```python
from build123d import *

# Parameters (mm, degrees)
SKETCH1_W                = 127
SKETCH1_H                = 127
SKETCH1_R                = 38.1
BOSS_EXTRUDE1_DEPTH      = 76.2
SKETCH2_R                = 6.35
CUT_EXTRUDE1_DEPTH       = 25.4
SKETCH3_R                = 63.5
SKETCH3_R_2              = 38.1
BOSS_EXTRUDE2_DEPTH      = 12.7
SKETCH4_W                = 12.7
SKETCH4_H                = 20.32
BOSS_EXTRUDE3_DEPTH      = 25.4
FILLET1_R                = 2.54
FILLET1_OF_MIRROR2_R     = 2.54
SKETCH5_W                = 76.2
SKETCH5_H                = 50.8
CUT_EXTRUDE3_DEPTH       = 10.16
FILLET2_R                = 7.62
SKETCH6_R                = 38.1
SKETCH6_R_2              = 31.75
BOSS_EXTRUDE4_DEPTH      = 25.4
BOSS_EXTRUDE4_DEPTH_BACK = 25.4


with BuildPart() as part:
    # Sketch1 → Boss-Extrude1 (new body)
    with BuildSketch(Plane(origin=(0, 0, 0), x_dir=(1, 0, 0), z_dir=(0, 1, 0))):
        Rectangle(SKETCH1_W, SKETCH1_H)
        Circle(SKETCH1_R, mode=Mode.SUBTRACT)
    extrude(amount=BOSS_EXTRUDE1_DEPTH)

    # Sketch2 → Cut-Extrude1 (cut)
    with BuildSketch(Plane.ZY.offset(63.5)):
        with Locations((-44.45, 57.15)):
            Circle(SKETCH2_R)
        with Locations((-44.45, 19.05)):
            Circle(SKETCH2_R)
        with Locations((44.45, 57.15)):
            Circle(SKETCH2_R)
        with Locations((44.45, 19.05)):
            Circle(SKETCH2_R)
    cut_extrude1 = extrude(amount=-CUT_EXTRUDE1_DEPTH, mode=Mode.SUBTRACT)

    # Mirror1: Cut-Extrude1 across plane
    add(cut_extrude1.mirror(Plane(origin=(0, 0, 0), x_dir=(0, 0, 1), z_dir=(1, 0, 0))), mode=Mode.SUBTRACT)

    # Sketch3 → Boss-Extrude2 (add)
    with BuildSketch(Plane.XZ):
        Circle(SKETCH3_R)
        Circle(SKETCH3_R_2, mode=Mode.SUBTRACT)
    extrude(amount=BOSS_EXTRUDE2_DEPTH)

    # Sketch4 → Boss-Extrude3 (add)
    with BuildSketch(Plane.XY.offset(63.5)):
        with Locations((-69.85, 38.1)):
            Rectangle(SKETCH4_W, SKETCH4_H)
        with Locations((69.85, 38.1)):
            Rectangle(SKETCH4_W, SKETCH4_H)
    boss_extrude3 = extrude(amount=-BOSS_EXTRUDE3_DEPTH)

    # Fillet1
    fillet1_edges = [part.edges().sort_by_distance(p)[0] for p in [
        (-69.85, 27.94, 38.1),
        (-69.85, 48.26, 38.1),
        (-69.85, 48.26, 63.5),
        (-69.85, 27.94, 63.5),
        (69.85, 48.26, 38.1),
        (69.85, 27.94, 38.1),
        (69.85, 27.94, 63.5),
        (69.85, 48.26, 63.5),
    ]]
    fillet(fillet1_edges, radius=FILLET1_R)

    # Mirror2: Boss-Extrude3 across plane
    add(boss_extrude3.mirror(Plane.XY))

    # Fillet1 of Mirror2
    fillet1_of_mirror2_edges = [part.edges().sort_by_distance(p)[0] for p in [
        (-69.85, 27.94, -38.1),
        (-69.85, 48.26, -38.1),
        (-69.85, 48.26, -63.5),
        (-69.85, 27.94, -63.5),
        (69.85, 48.26, -38.1),
        (69.85, 27.94, -38.1),
        (69.85, 27.94, -63.5),
        (69.85, 48.26, -63.5),
    ]]
    fillet(fillet1_of_mirror2_edges, radius=FILLET1_OF_MIRROR2_R)

    # Sketch5 → Cut-Extrude3 (cut)
    with BuildSketch(Plane(origin=(0, 0, 63.5), x_dir=(-1, 0, 0), z_dir=(0, 0, -1))):
        with Locations((0, 38.1)):
            Rectangle(SKETCH5_W, SKETCH5_H)
    extrude(amount=CUT_EXTRUDE3_DEPTH, mode=Mode.SUBTRACT)

    # Fillet2
    fillet2_edges = [part.edges().sort_by_distance(p)[0] for p in [
        (38.1, 63.5, 58.42),
        (38.1, 12.7, 58.42),
        (-38.1, 12.7, 58.42),
        (-38.1, 63.5, 58.42),
    ]]
    fillet(fillet2_edges, radius=FILLET2_R)

    # Sketch6 → Boss-Extrude4 (add, two sides)
    with BuildSketch(Plane(origin=(0, 31.75, 0), x_dir=(-1, 0, 0), z_dir=(0, -1, 0))) as boss_extrude4_sk:
        Circle(SKETCH6_R)
        Circle(SKETCH6_R_2, mode=Mode.SUBTRACT)
    extrude(amount=BOSS_EXTRUDE4_DEPTH)
    extrude(boss_extrude4_sk.sketch, amount=-BOSS_EXTRUDE4_DEPTH_BACK)


solid = part.part
```
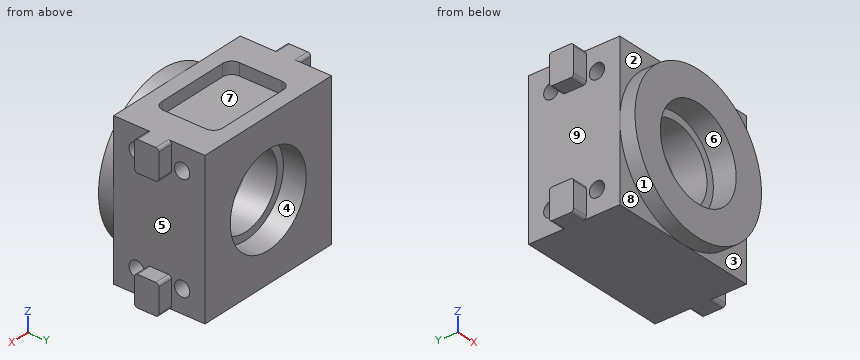
Check sheet for the modelled part. Datum: model origin and axes. Units: mm. Face numbers are marked on the shaded views. A direction names the side the tool comes from. Coordinates: 2 decimals unless noted, no trailing zeros. Loops run counter-clockwise (first coordinate to the right, second up) from the corner with the lowest first, then second, coordinate; pieces in that order, holes last. Notation, with made-up numbers: M -1.5,84.5 L 52.5,84.5 A23 cw 52.5,94.5 Z; hole C 4,-6.5 d4. An arc over 180 degrees is marked long. Answer as a JSON object with one key per item and string values.
1. Sectioned sample at D-D on x = -40.5. Record the cut outline in (y, z), and give its area (3 significant figures).
Outcome:
{"outline": "M -12.7,-48.91 L 0,-48.91 L 0,-63.5 L 76.2,-63.5 L 76.2,63.5 L 0,63.5 L 0,48.91 L -12.7,48.91 Z; hole C 19.05,-44.45 d12.7; hole C 19.05,44.45 d12.7; hole C 57.15,-44.45 d12.7; hole C 57.15,44.45 d12.7", "area": "10,400 mm²"}
2. Access from +Z, -Z, +X, -X, +Y, -Y to the whole of each face (thin tool, end or side, straight path). Record for the marked faces 1, 2, 3, 4 and 5.
Outcome:
{"face 1": "-Y", "face 2": "+Z, -X, -Y", "face 3": "-Z, +X, -Y", "face 4": "+Y", "face 5": "+X"}
3. Sectioned sample at A-A on z = -12. Record the cut outline in (x, y), and give its area (3 significant figures).
Outcome:
{"outline": "M -63.5,0 L -62.36,0 L -62.36,-12.7 L -36.16,-12.7 L -36.16,6.35 L -29.39,6.35 L -29.39,57.15 L -36.16,57.15 L -36.16,76.2 L -63.5,76.2 Z; M 29.39,6.35 L 36.16,6.35 L 36.16,-12.7 L 62.36,-12.7 L 62.36,0 L 63.5,0 L 63.5,76.2 L 36.16,76.2 L 36.16,57.15 L 29.39,57.15 Z", "area": "5,520 mm²"}
4. Sectioned sample at B-B on x = 44.5. Record the cut outline in (y, z), and give its area (3 significant figures).
Outcome:
{"outline": "M -12.7,-45.3 L 0,-45.3 L 0,-63.5 L 76.2,-63.5 L 76.2,63.5 L 0,63.5 L 0,45.3 L -12.7,45.3 Z; hole C 19.05,-44.45 d12.7; hole C 19.05,44.45 d12.7; hole C 57.15,-44.45 d12.7; hole C 57.15,44.45 d12.7", "area": "10,300 mm²"}
5. Scan lines: L1, parallel to Y at x = -46.75, z = -44.45; L2, parallel to Z at x = -49, y = 19; L3, parallel to X at y = 50, z = 0. Record each from-to range of solid material in increasing order. Write a range as from..to.
Outcome:
{"L1": "0..12.7, 25.4..50.8, 63.5..76.2", "L2": "-63.5..-50.8, -38.1..38.1, 50.8..63.5", "L3": "-63.5..-31.75, 31.75..63.5"}
6. Release check for a two-part mould opening along Z. For the marked faces 6, 7, 8 and 9 record: pulls with the +Z half, pulls with the -Z half, needs draft (parallel to the pull), parting line crosses it, or undercut.
Outcome:
{"face 6": "undercut", "face 7": "pulls with the +Z half", "face 8": "needs draft", "face 9": "undercut"}
7. Depth check by flat-ended pin: P1, Ø7.5, axis at y = 57.15, z = 44.45, coming from the +X side; P2, Ø1, axis at y = 59, z = 7, coming from the -X side; P3, Ø6.5, axis at x = -69.5, z = 55, coming from the -Y side. Enter the tip coordinate at first touch or a pass-through.
Outcome:
{"P1": "x = 38.1", "P2": "x = -63.5", "P3": "y = 27.94"}
